```python
from build123d import *

# Parameters (mm, degrees)
SKETCH1_W           = 406.4
SKETCH1_H           = 304.8
BOSS_EXTRUDE1_DEPTH = 4.7625
SKETCH2_R           = 16.51
SKETCH2_R_2         = 2.778125
SKETCH2_W           = 25.4
SKETCH2_H           = 101.6
CUT_EXTRUDE1_DEPTH  = 6.35


with BuildPart() as part:
    # Sketch1 → Boss-Extrude1 (new body)
    with BuildSketch(Plane(origin=(0, 0, 0), x_dir=(1, 0, 0), z_dir=(0, 1, 0))):
        with Locations((203.2, 152.4)):
            Rectangle(SKETCH1_W, SKETCH1_H)
    extrude(amount=BOSS_EXTRUDE1_DEPTH)

    # Sketch2 → Cut-Extrude1 (cut)
    with BuildSketch(Plane(origin=(0, 4.7625, 0), x_dir=(1, 0, 0), z_dir=(0, 1, 0))):
        with Locations(Location((57.15, 260.35, 0), (0, 0, 270))):
            Circle(SKETCH2_R)
        with Locations(Location((85.725, 260.35, 0), (0, 0, 270))):
            Circle(SKETCH2_R_2)
        with Locations(Location((28.575, 260.35, 0), (0, 0, 270))):
            Circle(SKETCH2_R_2)
        with Locations(Location((377.825, 260.35, 0), (0, 0, 90))):
            Circle(SKETCH2_R_2)
        with Locations(Location((320.675, 260.35, 0), (0, 0, 90))):
            Circle(SKETCH2_R_2)
        with Locations(Location((349.25, 260.35, 0), (0, 0, 90))):
            Circle(SKETCH2_R)
        with Locations((31.75, 69.85)):
            Rectangle(SKETCH2_W, SKETCH2_H)
        with Locations((374.65, 69.85)):
            Rectangle(SKETCH2_W, SKETCH2_H)
    extrude(amount=-CUT_EXTRUDE1_DEPTH, mode=Mode.SUBTRACT)


solid = part.part
```
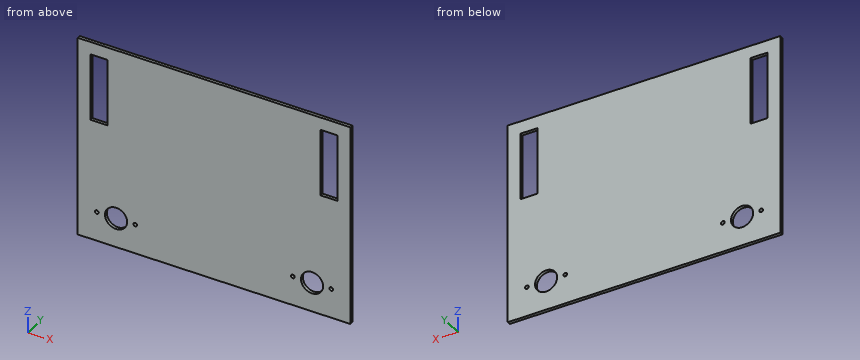
For this review, take the finished solid that the model builds, in its own axes (mm). Coordinates: 2 decimals unless noted, no trailing zeros. Loops run counter-clockwise (first coordinate to the right, second up) from the corner with the lowest first, then second, coordinate; pieces in that order, holes last.
1. Add section C-C, the plane y = 2.8. Count the separate pieces of the cut face and the enclosed holes in it, then the cut area to 3 significant figures.
2. Add section D-D, the plane x = 345. Give the boundary of the cut face in (y, z), then the cut area to 3 significant figures.
3. Add section A-A, the plane z = -71.5. Give the boundary of the cut face in (x, y), then the cut area to 3 significant figures.
4. For line 1 (X direction, y = 0.65, z = -69.5); line 2 (Z direction, x = 28.5, y = 4.6); line 3 (Z direction, x = 369.5, y = 0.8), list the stretches that pass through material, from the lowest coordinate up.
5. Add section B-B, the plane x = 57.15. Give the boundary of the cut face in (y, z).
Result:
1. separate pieces: 1
1. enclosed holes: 8
1. area: 117,000 mm2
2. outline: (0, -304.8) - (4.76, -304.8) - (4.76, -276.3) - (0, -276.3) - close; (0, -244.4) - (4.76, -244.4) - (4.76, 0) - (0, 0) - close
2. area: 1,300 mm2
3. outline: (0, 0) - (19.05, 0) - (19.05, 4.76) - (0, 4.76) - close; (44.45, 0) - (361.95, 0) - (361.95, 4.76) - (44.45, 4.76) - close; (387.35, 0) - (406.4, 0) - (406.4, 4.76) - (387.35, 4.76) - close
3. area: 1,690 mm2
4. line 1: x = 0 to 19.05, 44.45 to 361.95, 387.35 to 406.4
4. line 2: z = -304.8 to -263.13, -257.57 to -120.65, -19.05 to 0
4. line 3: z = -304.8 to -120.65, -19.05 to 0
5. outline: (0, -304.8) - (4.76, -304.8) - (4.76, -276.86) - (0, -276.86) - close; (0, -243.84) - (4.76, -243.84) - (4.76, 0) - (0, 0) - close
